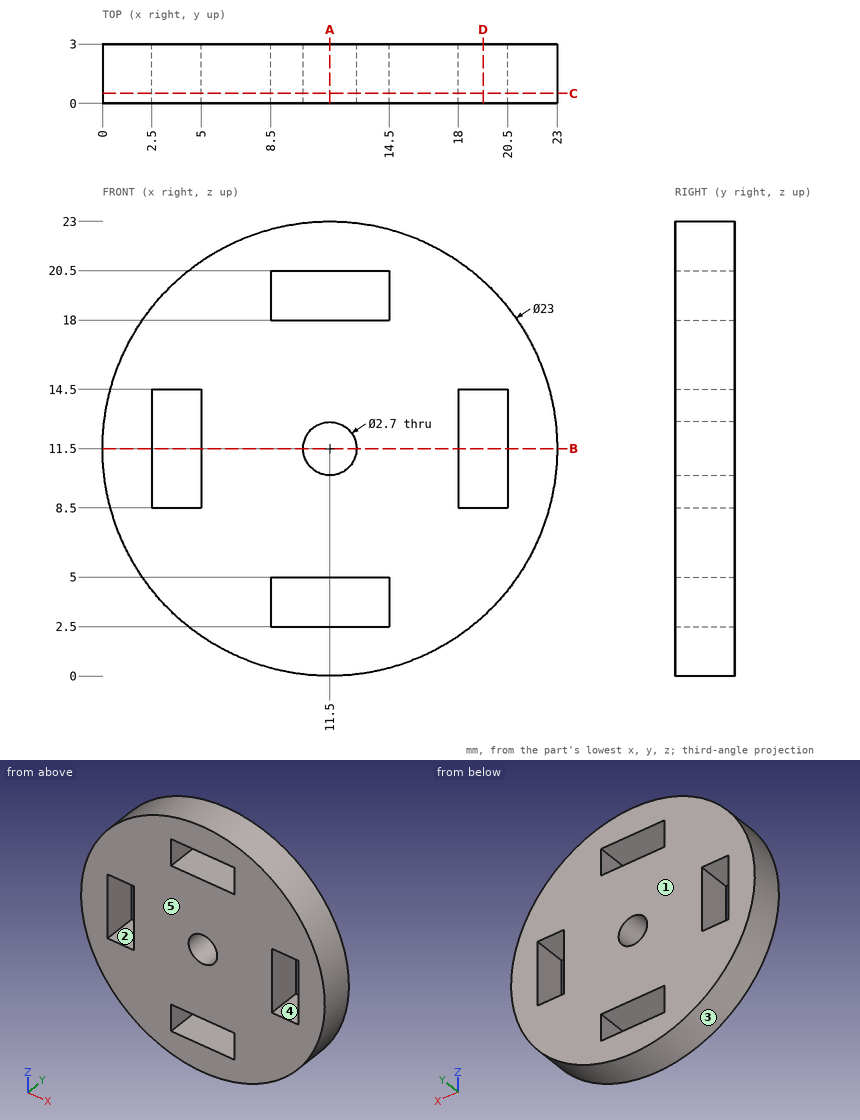
Could you check a few things on this drawing? It's one solid part, dimensions in mm from its lowest x, y, z. A direction names the side the tool comes from. Coordinates: 2 decimals unless noted, no trailing zeros. Order: outer loops, then holes, each group sorted by start corner. A loop starts at its lowest first (then second) coordinate and runs counter-clockwise, first axis right, second up. Notation, with made-up numbers: (16, -36) - (59, -36) arc R24 ccw to (59, -20) - close; hole circle Ø7 at (83.25, 8). An arc over 180 degrees is marked (long way). One line per question, with ' | ' between items. Start each with the question number.
1. If we section it at D-D (x = 19.25): Write out the boundary of the cut face in (y, z), and give its area (3 significant figures).
2. I'm going to push flat-ended pins straight in: pin 1 Ø1.5 at (y, z) = (2.5, 13) entering from -X; pin 2 Ø0.8 at (y, z) = (1, 19) entering from +X. Where does each tip first touch, or does it pass through?
3. If we mould it in two halves opening along X, with no side actions, what happens to the marked faces 1, 2 and 3? For each: released by +X, released by -X, zero draft, split by the parting line, or undercut.
4. Which directions (+Z, -Z, +X, -X, +Y, -Y) give clear straight access to the entire face, cutting with the end or side of a thin tool? Please do the marked faces 4 and 5.
5. If we section it at C-C (y = 0.5): Write out the boundary of the cut face in (x, z), and give its area (3 significant figures).
6. If we section it at A-A (x = 11.5): Write out the boundary of the cut face in (y, z), and give its area (3 significant figures).
7. If we section it at B-B (z = 11.5): Write out the boundary of the cut face in (x, y).
8. Please list where these lines run through material, in increasing order: line 1 along X through (y, z) = (1.45, 11.5); line 2 along Z through (x, y) = (10, 0.8); line 3 along Z through (x, y) = (12, 1.65). Write a range as [from, to].
Model answer:
1) outline: (0, 3) - (3, 3) - (3, 8.5) - (0, 8.5) - close; (0, 14.5) - (3, 14.5) - (3, 20) - (0, 20) - close | area: 33.0 mm²
2) pin 1: stops at x = 0.02 | pin 2: stops at x = 20.55
3) face 1: zero draft | face 2: undercut | face 3: split by the parting line
4) face 4: +Y, -Y | face 5: +Z, -Z, +X, -X, -Y
5) outline: circle Ø23 at (11.5, 11.5); hole (2.5, 8.5) - (5, 8.5) - (5, 14.5) - (2.5, 14.5) - close; hole (8.5, 2.5) - (14.5, 2.5) - (14.5, 5) - (8.5, 5) - close; hole (8.5, 18) - (14.5, 18) - (14.5, 20.5) - (8.5, 20.5) - close; hole circle Ø2.7 at (11.5, 11.5); hole (18, 8.5) - (20.5, 8.5) - (20.5, 14.5) - (18, 14.5) - close | area: 350 mm²
6) outline: (0, 0) - (3, 0) - (3, 2.5) - (0, 2.5) - close; (0, 5) - (3, 5) - (3, 10.15) - (0, 10.15) - close; (0, 12.85) - (3, 12.85) - (3, 18) - (0, 18) - close; (0, 20.5) - (3, 20.5) - (3, 23) - (0, 23) - close | area: 45.9 mm²
7) outline: (0, 0) - (2.5, 0) - (2.5, 3) - (0, 3) - close; (5, 0) - (10.15, 0) - (10.15, 3) - (5, 3) - close; (12.85, 0) - (18, 0) - (18, 3) - (12.85, 3) - close; (20.5, 0) - (23, 0) - (23, 3) - (20.5, 3) - close
8) line 1: x = [0, 2.5], [5, 10.15], [12.85, 18], [20.5, 23] | line 2: z = [0.1, 2.5], [5, 18], [20.5, 22.9] | line 3: z = [0.01, 2.5], [5, 10.25], [12.75, 18], [20.5, 22.99]
